from build123d import *

# Parameters (mm, degrees)
F1_DEPTH = 5
F2_R     = 8.5
F3_R     = 4
F4_R     = 9.5
F5_R     = 1


with BuildPart() as f1:
    # F0 (on Front) → F1 (new body)
    with BuildSketch(Plane.XZ):
        Polygon((5, 110.628678), (0, 110.628678), (0, 0), (35.341783, 3.714571), (33.355742, 22.610487), (23.907784, 21.617467), (24.900804, 12.169509), (15.452846, 11.176488), align=None)
    extrude(amount=F1_DEPTH)

    # F2
    f2_edges = [f1.edges().sort_by_distance(p)[0] for p in [
        (33.355742, -2.5, 22.610487),
    ]]
    fillet(f2_edges, radius=F2_R)

    # F3
    f3_edges = [f1.edges().sort_by_distance(p)[0] for p in [
        (15.452846, -2.5, 11.176488),
    ]]
    fillet(f3_edges, radius=F3_R)

    # F4
    f4_edges = [f1.edges().sort_by_distance(p)[0] for p in [
        (35.341783, -2.5, 3.714571),
    ]]
    fillet(f4_edges, radius=F4_R)

    # F5
    f5_edges = [f1.edges().sort_by_distance(p)[0] for p in [
        (24.900804, -2.5, 12.169509),
    ]]
    fillet(f5_edges, radius=F5_R)


solid = f1.part
CAD build for the part. Positions are in the model's coordinates, mm. A direction names the side the tool comes from. Round coordinates to 2 decimals unless told otherwise and drop trailing zeros. Write each loop counter-clockwise with the first axis right and the second up, starting at its lowest first coordinate (ties: lowest second). Pieces come first, ordered by that corner, then holes.
(1) 3-axis set-ups, long thin cutter, end or side, ignore diameter. For faces 1 (the face through (0, -2, 56)), 2 (the face through (21.7, -2.465, 11.833)): which of +Z, -Z, +X, -X, +Y, -Y reach the whole face in a straight line?
(2) Mould opens along X. For faces 3 (the face through (24.346, -2.465, 17.45)), 4 (the face through (12.766, -2.465, 1.342)), 5 (the face through (9, -5, 44)) say: pulls with the +X half, pulls with the -X half, needs draft (parallel to the pull), parting line crosses it, or undercut.
(3) Slice it at B-B, the plane z = 16.5. Write the cut outline in (x, y), and give its area (3 significant figures).
(4) Slice it at C-C, the plane x = 14. Write the cut outline in (y, z).
(5) Drop flat-ended pins along their axis: P1, Ø8, axis at x = 25.5, z = 25, coming from the -Y side; P2, Ø1, axis at x = 8, y = -2.5, coming from the -Z side; P3, Ø1, axis at x = 24, y = -2, coming from the -Z side; P4, Ø3, axis at x = 11.5, y = -2.5, coming from the -Z side. Give the stop position or say it passes through.
(6) Probe line 1 along Z through (x, y) = (2.5, -4); line 2 along Z through (x, y) = (26, -3.55); line 3 along X through (y, z) = (-1.4, 20). List the from-to ranges inside material, lowest first.
(7) Slice it at A-A, the plane y = -1.55. Write the cut outline in (x, z).
(8) Slice it at D-D, the plane z = 77. Write the cut outline in (x, y), and give its area (3 significant figures).
From the geometry:
1. face 1: +Z, -Z, -X, +Y, -Y
1. face 2: +Z, +Y, -Y
2. face 3: undercut
2. face 4: pulls with the +X half
2. face 5: needs draft
3. outline: (0, -5) - (14.89, -5) - (14.89, 0) - (0, 0) - close; (24.45, -5) - (33.65, -5) - (33.65, 0) - (24.45, 0) - close
3. area: 121 mm2
4. outline: (-5, 1.47) - (0, 1.47) - (0, 25) - (-5, 25) - close
5. P1: stops at y = -5
5. P2: stops at z = 0.79
5. P3: stops at z = 2.47
5. P4: stops at z = 1.05
6. line 1: z = 0.26 to 110.63
6. line 2: z = 2.73 to 21.77
6. line 3: x = 0 to 14.53, 24.08 to 30.98
7. outline: (0, 0) - (25.89, 2.72) arc R9.5 ccw to (34.35, 13.16) - (34.24, 14.16) arc R8.5 ccw to (24.9, 21.72) - (23.91, 21.62) - (24.8, 13.16) arc R1 cw to (23.91, 12.06) - (19.43, 11.59) arc R4 cw to (15.03, 15.15) - (5, 110.63) - (0, 110.63) - close
8. outline: (0, -5) - (8.53, -5) - (8.53, 0) - (0, 0) - close
8. area: 42.7 mm2
